Autodesk Inventor part; units mm, degrees
ref_plane "MSC_PF1" through (0, 0, 0) normal (1, 0, 0) x (0, 1, 0)
ref_plane "MSC_PT1" through (0, 0, 0) normal (0, 0, 1) x (1, 0, 0)
ref_plane "YZ Plane" through (0, 0, 0) normal (1, 0, 0) x (0, 1, 0)
sketch "Sketch7" plane through (0, 0, 0) normal (0, 0, 1) x (1, 0, 0)
  circle A0 centre (0, 0) radius 3.9688 construction
  line L0 (-3.9688, -2.2914) -> (-3.9688, 2.2914)
  line L1 (-3.9688, 2.2914) -> (0, 4.5827)
  line L2 (0, 4.5827) -> (3.9688, 2.2914)
  line L3 (3.9688, 2.2914) -> (3.9688, -2.2914)
  line L4 (3.9688, -2.2914) -> (0, -4.5827)
  line L5 (0, -4.5827) -> (-3.9688, -2.2914)
  dimension "d40" = 7.9375
extrude "Extrusion1" add sketch "Sketch7" against normal blind 2.8956
sketch "Sketch11" plane through (0, 0, 0) normal (0, 0, 1) x (1, 0, 0)
  line L0 (0, 4.5827) -> (3.9688, 2.2914)
  line L1 (-3.9688, 2.2914) -> (0, 4.5827)
  line L2 (-3.9688, 2.2914) -> (3.9688, -2.2914) construction
  line L3 (-3.9688, -2.2914) -> (3.9688, 2.2914) construction
  point P0 (0, 0)
hole "Hole1" at (0, 0, 0) direction (0, 0, -1) diameter 2.6416 end through all
chamfer "Chamfer1" distance 0.0156 angle 45 2 edges at (0, 1.3208, 0) (0, 1.3208, -2.8956)
sketch "Sketch9" plane through (0, 0, 0) normal (1, 0, 0) x (0, 1, 0)
  line L0 (-4.5827, -2.5411) -> (-4.5827, -2.8956)
  line L1 (-4.5827, -2.8956) -> (-3.9688, -2.8956)
  line L2 (-3.9688, -2.8956) -> (-4.5827, -2.5411)
  line L3 (0, -2.9665) -> (0, -2.4702)
  line L4 (-4.5827, -2.8956) -> (-2.2914, -2.8956)
  dimension "d38" = 7.9375
  dimension "d41" = 150
revolve "Revolution1" cut sketch "Sketch9" angle 360 about axis through (0, 0, -10) along (0, 0, 1)
sketch "Sketch10" plane through (0, 0, 0) normal (1, 0, 0) x (0, 1, 0)
  line L0 (-4.5827, -0.3545) -> (-4.5827, 0)
  line L1 (-4.5827, 0) -> (-3.9688, 0)
  line L2 (-3.9688, 0) -> (-4.5827, -0.3545)
  line L3 (0, -0.4254) -> (0, 0.0709)
  line L4 (-2.2914, 0) -> (-4.5827, 0)
  dimension "d45" = 7.9375
  dimension "d46" = 150
revolve "Revolution2" cut sketch "Sketch10" angle 360 about axis through (0, 0, -10) along (0, 0, 1)
ref_plane "MSC_PF1" through (0, 0, 0) normal (1, 0, 0) x (0, 1, 0)
ref_plane "MSC_PT1" through (0, 0, 0) normal (0, 0, 1) x (1, 0, 0)
equation "\"d38\" = Fbas"
equation "\"d40\" = Fbas"
equation "\"d29\" = Hbas"
equation "\"d63\" = 0.5 * PTC"
equation "\"d45\" = Fbas"
equation "\"Fbas\" = 7.9375"
equation "\"Hbas\" = 2.8956"
equation "\"NND\" = 3.5052"
equation "\"THREADDIA\" = NND"
properties part number "ASME B18.6.3 - 6-32" material "Steel, Mild"
Source: CAD feature listing. Evaluate the final solid. Frame: model axes, mm. Give positions to 0.01 mm unless a question says otherwise; leave off trailing zeros. Write each loop counter-clockwise with the first axis right and the second up, starting at its lowest first coordinate (ties: lowest second). Pieces come first, ordered by that corner, then holes. Notation, with made-up numbers: M 10,-14.5 L 50,-14.5 A26 ccw 50,23.5 Z; hole C 31,-21.75 d11. An arc over 180 degrees is marked long. Return JSON: item names as keys, results as strings. Group by question number.
1) Material intervals for line 1 along X through (y, z) = (0, -1.25); line 2 along X through (y, z) = (3.25, -2.45); line 3 along Z through (x, y) = (-3.5, 2), sorted ascending. Write a range as [from, to].
2) Pull-direction query (X, two-part tool) for faces 1 (the face through (3.561, 2.068, -0.086)), 2 (the face through (0.8, 1.05, -1.47)), 3 (the face through (-2.01, 3.42, -1.43)); classes: pulls with the +X half, pulls with the -X half, needs draft (parallel to the pull), parting line crosses it, or undercut.
3) Pin query (flat end, axial travel): P1, Ø3, axis at x = -2, y = -1, coming from the +Z side. Return the tip coordinate at first contact, or that it passes through.
4) Cut plane A-A, the plane z = -2.1. Output: boundary loops of the cut face in (x, y), plus the area to 3 significant figures.
Recorded:
{
 "1": {"line 1": "x = [-3.97, -1.32], [1.32, 3.97]", "line 2": "x = [-2.31, 2.31]", "line 3": "z = [-2.86, -0.04]"},
 "2": {"face 1": "pulls with the +X half", "face 2": "undercut", "face 3": "pulls with the -X half"},
 "3": {"P1": "stops at z = 0"},
 "4": {"outline": "M -3.97,-2.29 L 0,-4.58 L 3.97,-2.29 L 3.97,2.29 L 0,4.58 L -3.97,2.29 Z; hole C 0,0 d2.64", "area": "49.1 mm²"}
}
